Autodesk Inventor part; units mm, degrees
ref_plane "YZ Plane" through (0, 0, 0) normal (1, 0, 0) x (0, 1, 0)
ref_plane "XZ Plane" through (0, 0, 0) normal (0, 1, 0) x (-1, 0, 0)
ref_plane "XY Plane" through (0, 0, 0) normal (0, 0, 1) x (1, 0, 0)
sketch "Sketch1" plane through (0, 0, 0) normal (0, 0, 1) x (1, 0, 0)
  line L0 (-3.175, -3.175) -> (3.175, -3.175)
  line L1 (3.175, -3.175) -> (3.175, 3.175)
  line L2 (3.175, 3.175) -> (-3.175, 3.175)
  line L3 (-3.175, 3.175) -> (-3.175, -3.175)
  line L4 (-3.175, -3.175) -> (3.175, 3.175) construction
  line L5 (3.175, -3.175) -> (-3.175, 3.175) construction
  point P0 (0, 0)
  dimension "d0" = 6.35
  dimension "d1" = 6.35
extrude "Extrusion1" add sketch "Sketch1" along normal blind 15.875
sketch "Sketch2" plane through (-3.175, 3.175, 0) normal (0, 1, 0) x (1, 0, 0)
  line L0 (3.175, 0) -> (3.175, -15.875) construction
  line L1 (6.35, -15.875) -> (0, -15.875)
  circle A0 centre (3.175, -7.9375) radius 1.7526
  circle A1 centre (3.175, -41.275) radius 1.4493 construction
  line L2 (6.35, 0) -> (0, 0)
  dimension "d4" = 3.5052
  dimension "d13" = 7.9375
extrude "Extrusion2" cut sketch "Sketch2" against normal through all
sketch "Sketch3" plane through (3.175, -3.175, 0) normal (1, 0, 0) x (0, 0, -1)
  line L0 (0, 3.175) -> (-15.875, 3.175) construction
  line L1 (-15.875, 0) -> (-15.875, 6.35)
  circle A0 centre (-12.7, 3.175) radius 1.7526
  circle A1 centre (-3.175, 3.175) radius 1.7526
  circle A2 centre (6.35, 3.175) radius 1.7526
  circle A3 centre (15.875, 3.175) radius 1.7526
  dimension "d16" = 3.5052
  dimension "d17" = 3.175
  dimension "d20" = 9.525
extrude "Extrusion3" cut sketch "Sketch3" against normal through all
chamfer "Chamfer1" distance 0.1 angle 45 4 edges at (-3.175, 3.175, 7.9375) (3.175, 3.175, 7.9375) (3.175, -3.175, 7.9375) (-3.175, -3.175, 7.9375)
properties part number "Nut Strip" material "Aluminum 6061"
Can you work these out from the model? Positions are in its coordinate system, mm. Round coordinates to 2 decimals unless told otherwise and drop trailing zeros. Order: outer loops, then holes, each group sorted by start corner. A loop starts at its lowest first (then second) coordinate and runs counter-clockwise, first axis right, second up. Notation, with made-up numbers: M 86.25,6 L 142.25,6 A33 ccw 142.25,36 Z; hole C 87.5,-2 d9. An arc over 180 degrees is marked long. Use a Markdown table: item, result.
1) If we mould it in two halves opening along Y, with no side actions, what happens to faces 1 (the face through (-3.175, 0, 8)), 2 (the face through (0.04, 0.08, 14.45)), 3 (the face through (0, 3.175, 6)), 4 (the face through (0.044, 0.526, 1.503))? For each: +Y half, -Y half, draft (parallel to the pull), parting line (faces both ways), or undercut.
Geometry says:
| item | result |
|---|---|
| face 1 | draft |
| face 2 | undercut |
| face 3 | +Y half |
| face 4 | undercut |
2) If I drill on line 1 along Z through (x, y) = (-1.25, 0.75) (3 decimals); line 2 along Z through (x, y) = (0, 0.5) (3 decimals); line 3 along Y through (x, z) = (0.5, 12.7) (3 decimals), over which ranges is the centre line in solid material (lowest first)?
Geometry says:
| item | result |
|---|---|
| line 1 | z = 0 to 1.591, 4.759 to 6.709, 9.166 to 11.116, 14.284 to 15.875 |
| line 2 | z = 0 to 1.495, 4.855 to 6.185, 9.69 to 11.02, 14.38 to 15.875 |
| line 3 | y = -3.175 to -1.753, 1.753 to 3.175 |
3) Imagine slicing it at D-D (x = -2.5). List the corners of the cut face in (y, z) for me (3 decimals).
Geometry says:
| item | result |
|---|---|
| outline | M -3.175,0 L 3.175,0 L 3.175,15.875 L -3.175,15.875 Z; hole C 0,3.175 d3.505; hole C 0,12.7 d3.505 |
4) Imagine slicing it at A-A (x = 0). List the corners of the cut face in (y, z) for me (3 decimals), then the cut area to 3 significant figures.
Geometry says:
| item | result |
|---|---|
| outline | M -3.175,0 L 3.175,0 L 3.175,6.185 L -3.175,6.185 Z; M -3.175,9.69 L 3.175,9.69 L 3.175,15.875 L -3.175,15.875 Z; hole C 0,3.175 d3.505; hole C 0,12.7 d3.505 |
| area | 59.2 mm² |
5) Imagine slicing it at B-B (z = 12.7). List the corners of the cut face in (x, y) for me (3 decimals).
Geometry says:
| item | result |
|---|---|
| outline | M -3.175,-3.075 L -3.075,-3.175 L 3.075,-3.175 L 3.175,-3.075 L 3.175,-1.753 L -3.175,-1.753 Z; M -3.175,1.753 L 3.175,1.753 L 3.175,3.075 L 3.075,3.175 L -3.075,3.175 L -3.175,3.075 Z |
6) Imagine slicing it at C-C (y = -0.5). List the corners of the cut face in (x, z) for me (1 decimal).
Geometry says:
| item | result |
|---|---|
| outline | M -3.2,0 L 3.2,0 L 3.2,1.5 L -3.2,1.5 Z; M -3.2,4.9 L 3.2,4.9 L 3.2,11 L -3.2,11 Z; M -3.2,14.4 L 3.2,14.4 L 3.2,15.9 L -3.2,15.9 Z; hole C 0,7.9 d3.5 |
